```python
from build123d import *

# Parameters (mm, degrees)
SKETCH1_R           = 3
BOSS_EXTRUDE1_DEPTH = 49.8


with BuildPart() as part:
    # Sketch1 → Boss-Extrude1 (new body)
    with BuildSketch(Plane(origin=(0, 0, 0), x_dir=(1, 0, 0), z_dir=(0, 1, 0))):
        Polygon((-149.99, -10), (43.99, -10), (53, -4.8), (53, 4.8), (43.99, 10), (-149.99, 10), (-159, 4.8), (-159, -4.8), align=None)
        with BuildLine():
            ThreePointArc((33.8348486, 8), (37.1814887, 6.190890255), (37.500909186, 2.400000045))
            ThreePointArc((37.500909186, 2.400000045), (37, 1e-09), (37.500909185, -2.400000042))
            ThreePointArc((37.500909185, -2.400000042), (37.181488707, -6.190890243), (33.834848625, -8))
            Line((33.834848625, -8), (14.165151315, -8))
            ThreePointArc((14.165151315, -8), (10.818511261, -6.190890195), (10.499090838, -2.399999991))
            ThreePointArc((10.499090838, -2.399999991), (11, -3e-09), (10.49909084, 2.399999985))
            ThreePointArc((10.49909084, 2.399999985), (10.81851128, 6.190890224), (14.165151391, 8))
            Line((14.165151391, 8), (33.8348486, 8))
        make_face(mode=Mode.SUBTRACT)
        with BuildLine():
            ThreePointArc((-0.499090895, 2.39999986), (-1, 1.1e-08), (-0.499090904, -2.399999839))
            ThreePointArc((-0.499090904, -2.399999839), (-0.818511236, -6.190890157), (-4.16515139, -8))
            Line((-4.16515139, -8), (-23.83484861, -8))
            ThreePointArc((-23.83484861, -8), (-27.181488692, -6.190890267), (-27.500909202, -2.400000081))
            ThreePointArc((-27.500909202, -2.400000081), (-27, -3.4e-08), (-27.500909174, 2.400000019))
            ThreePointArc((-27.500909174, 2.400000019), (-27.181488711, 6.190890238), (-23.83484861, 8))
            Line((-23.83484861, 8), (-4.165151415, 8))
            ThreePointArc((-4.165151415, 8), (-0.818511249, 6.190890177), (-0.499090895, 2.39999986))
        make_face(mode=Mode.SUBTRACT)
        with BuildLine():
            ThreePointArc((-38.499090754, -2.400000183), (-38.818511346, -6.190890325), (-42.165151417, -8))
            Line((-42.165151417, -8), (-51, -8))
            Line((-51, -8), (-51, 8))
            Line((-51, 8), (-42.165151363, 8))
            ThreePointArc((-42.165151363, 8), (-38.818511221, 6.190890134), (-38.499090914, 2.399999815))
            ThreePointArc((-38.499090914, 2.399999815), (-39, -2e-07), (-38.499090754, -2.400000183))
        make_face(mode=Mode.SUBTRACT)
        with BuildLine():
            Line((-55, 8), (-55, -8))
            Line((-55, -8), (-63.834848637, -8))
            ThreePointArc((-63.834848637, -8), (-67.181488771, -6.190890146), (-67.500909096, -2.39999984))
            ThreePointArc((-67.500909096, -2.39999984), (-67, 9e-08), (-67.500909168, 2.400000005))
            ThreePointArc((-67.500909168, 2.400000005), (-67.181488707, 6.190890244), (-63.834848583, 8))
            Line((-63.834848583, 8), (-55, 8))
        make_face(mode=Mode.SUBTRACT)
        with BuildLine():
            ThreePointArc((-78.499090904, 2.39999984), (-79, -1.79e-07), (-78.49909076, -2.400000169))
            ThreePointArc((-78.49909076, -2.400000169), (-78.818511334, -6.190890307), (-82.16515139, -8))
            Line((-82.16515139, -8), (-101.83484861, -8))
            ThreePointArc((-101.83484861, -8), (-105.181488717, -6.190890228), (-105.500909164, -2.399999996))
            ThreePointArc((-105.500909164, -2.399999996), (-105, 1.3e-08), (-105.500909175, 2.40000002))
            ThreePointArc((-105.500909175, 2.40000002), (-105.18148871, 6.190890239), (-101.83484861, 8))
            Line((-101.83484861, 8), (-82.16515139, 8))
            ThreePointArc((-82.16515139, 8), (-78.818511236, 6.190890157), (-78.499090904, 2.39999984))
        make_face(mode=Mode.SUBTRACT)
        with BuildLine():
            ThreePointArc((-116.499090787, 2.400000107), (-117, 5.5e-08), (-116.499090832, -2.400000005))
            ThreePointArc((-116.499090832, -2.400000005), (-116.818511285, -6.190890232), (-120.16515139, -8))
            Line((-120.16515139, -8), (-139.83484861, -8))
            ThreePointArc((-139.83484861, -8), (-143.181488722, -6.190890221), (-143.500909157, -2.39999998))
            ThreePointArc((-143.500909157, -2.39999998), (-143, 1.5e-08), (-143.500909169, 2.400000007))
            ThreePointArc((-143.500909169, 2.400000007), (-143.181488714, 6.190890233), (-139.83484861, 8))
            Line((-139.83484861, 8), (-120.16515139, 8))
            ThreePointArc((-120.16515139, 8), (-116.818511316, 6.190890279), (-116.499090787, 2.400000107))
        make_face(mode=Mode.SUBTRACT)
        with Locations(Location((-149, 0, 0), (0, 0, 270))):
            Circle(SKETCH1_R, mode=Mode.SUBTRACT)
        with Locations(Location((-73, 0, 0), (0, 0, 270))):
            Circle(SKETCH1_R, mode=Mode.SUBTRACT)
        with Locations(Location((-111, 0, 0), (0, 0, 270))):
            Circle(SKETCH1_R, mode=Mode.SUBTRACT)
        with Locations(Location((-33, 0, 0), (0, 0, 270))):
            Circle(SKETCH1_R, mode=Mode.SUBTRACT)
        with Locations(Location((5, 0, 0), (0, 0, 270))):
            Circle(SKETCH1_R, mode=Mode.SUBTRACT)
        with Locations(Location((43, 0, 0), (0, 0, 270))):
            Circle(SKETCH1_R, mode=Mode.SUBTRACT)
    extrude(amount=BOSS_EXTRUDE1_DEPTH)


solid = part.part
```
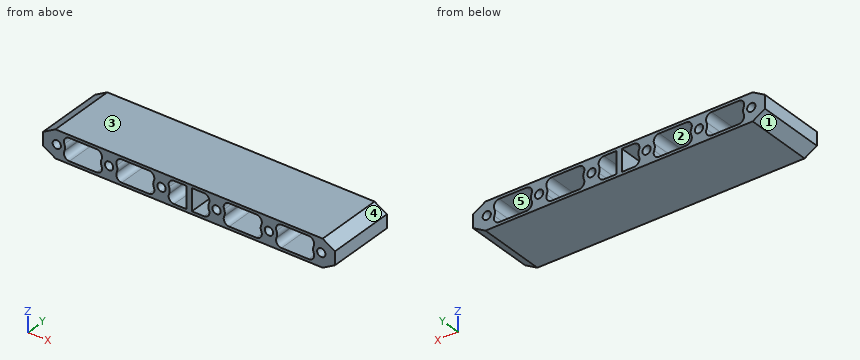
Here's how the part is built. I have some questions about the finished solid (model axes, mm). Face numbers are marked on the shaded views. A direction names the side the tool comes from. Coordinates: 2 decimals unless noted, no trailing zeros. Order: outer loops, then holes, each group sorted by start corner. A loop starts at its lowest first (then second) coordinate and runs counter-clockwise, first axis right, second up. Notation, with made-up numbers: (-22.5, -20.5) - (8.5, -20.5) arc R30 cw to (8.5, 18.5) - close; hole circle Ø10 at (19, -32). An arc over 180 degrees is marked (long way). One line per question, with ' | ' between items. Start each with the question number.
1. Please list where these lines run through material, in increasing order: line 1 along Z through (x, y) = (-20.5, 23); line 2 along Z through (x, y) = (-149, 14). Write a range as [from, to].
2. I'm going to push flat-ended pins straight in: pin 1 Ø3.5 at (x, z) = (-33, 0) entering from -Y; pin 2 Ø1 at (x, z) = (10.5, 3.5) entering from -Y. Where does each tip first touch, or does it pass through?
3. If we section it at B-B (z = 0): Give the number of separate pieces and of enclosed holes in the cut face, and give its area (3 significant figures).
4. Which directions (+Z, -Z, +X, -X, +Y, -Y) give clear straight access to the entire face, cutting with the end or side of a thin tool? Please do the marked faces 1 and 2.
5. If we section it at A-A (x = 5): Write out the boundary of the cut face in (y, z).
6. If we mould it in two halves opening along X, with no side actions, what happens to the marked faces 3, 4 and 5? For each: released by +X, released by -X, zero draft, split by the parting line, or undercut.
Model answer:
1) line 1: z = [-10, -8], [8, 10] | line 2: z = [-10, -3], [3, 10]
2) pin 1: passes through | pin 2: stops at y = 0
3) separate pieces: 13 | enclosed holes: 0 | area: 2,390 mm²
4) face 1: -Z, -X, +Y, -Y | face 2: +Y, -Y
5) outline: (0, -10) - (49.8, -10) - (49.8, -3) - (0, -3) - close; (0, 3) - (49.8, 3) - (49.8, 10) - (0, 10) - close
6) face 3: zero draft | face 4: released by +X | face 5: undercut
